Part print with two shaded views. Sizes in mm from the minimum x, y, z corner. Give positions to 0.01 mm unless a question says otherwise; leave off trailing zeros. Write each loop counter-clockwise with the first axis right and the second up, starting at its lowest first coordinate (ties: lowest second). Pieces come first, ordered by that corner, then holes. Notation, with made-up numbers: (-8.5, 74) -> (48.5, 74) arc R27 cw to (48.5, 105) -> close; hole circle Ø3 at (56.5, 49.25). An arc over 180 degrees is marked (long way). Answer as a JSON object with one key per item and string values.
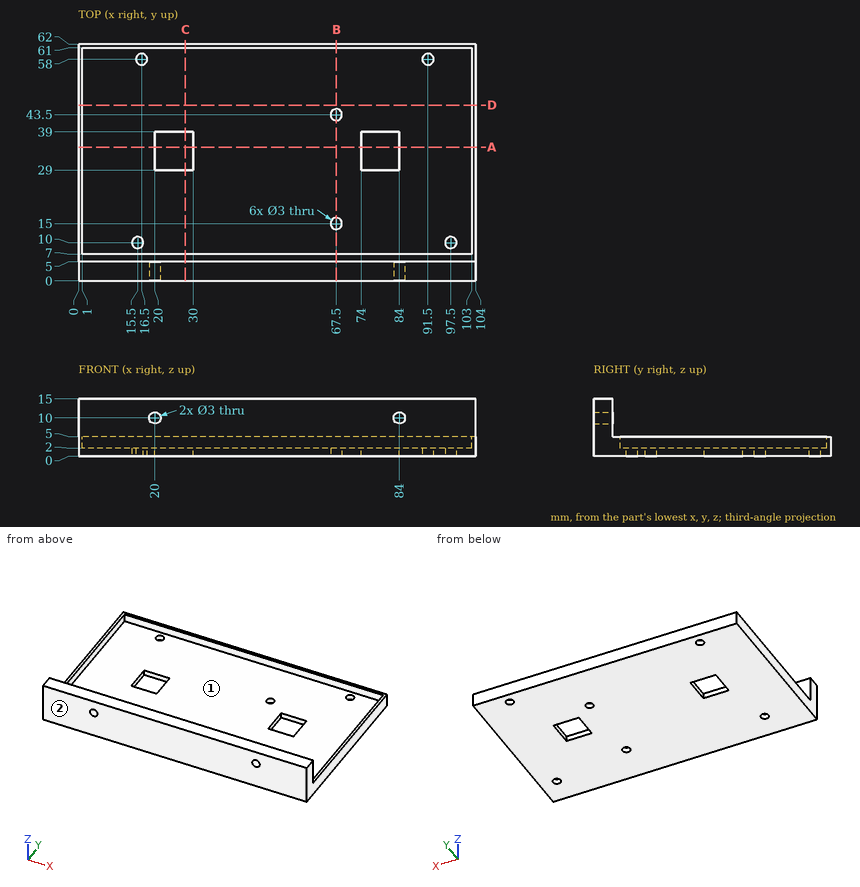
1) Slice it at C-C (x = 28). List the corners of the cut face in (y, z).
Model answer:
{"outline": "(0, 0) -> (29, 0) -> (29, 2) -> (7, 2) -> (7, 5) -> (5, 5) -> (5, 15) -> (0, 15) -> close; (39, 0) -> (62, 0) -> (62, 5) -> (61, 5) -> (61, 2) -> (39, 2) -> close"}
2) Wall check: probe 1 along Y at (x, z) = (67.5, 0.95); probe 2 along Z at (x, y) = (20, 1); probe 3 along X at (y, z) = (43.5, 0.9). Give the ranges that are in metal, low to high.
Model answer:
{"probe 1": "y = 0 to 13.5, 16.5 to 42, 45 to 62", "probe 2": "z = 0 to 8.5, 11.5 to 15", "probe 3": "x = 0 to 66, 69 to 104"}
3) Slice it at A-A (y = 35). List the corners of the cut face in (x, z), then the cut area to 3 significant figures.
Model answer:
{"outline": "(0, 0) -> (20, 0) -> (20, 2) -> (1, 2) -> (1, 5) -> (0, 5) -> close; (30, 0) -> (74, 0) -> (74, 2) -> (30, 2) -> close; (84, 0) -> (104, 0) -> (104, 5) -> (103, 5) -> (103, 2) -> (84, 2) -> close", "area": "174 mm2"}
4) Pin check, flat tips, straight feed: pin 1 (5 mm diameter, centred on x = 25, y = 8, fed in from +Z); pin 2 (3 mm diameter, centred on x = 39, z = 7, fed in from +Y); pin 3 (5 mm diameter, centred on x = 45.5, y = 26, fed in from +Z). Stop position of each tip, or through.
Model answer:
{"pin 1": "stops at z = 5", "pin 2": "stops at y = 5", "pin 3": "stops at z = 2"}
5) Slice it at B-B (x = 67.5). List the corners of the cut face in (y, z).
Model answer:
{"outline": "(0, 0) -> (13.5, 0) -> (13.5, 2) -> (7, 2) -> (7, 5) -> (5, 5) -> (5, 15) -> (0, 15) -> close; (16.5, 0) -> (42, 0) -> (42, 2) -> (16.5, 2) -> close; (45, 0) -> (62, 0) -> (62, 5) -> (61, 5) -> (61, 2) -> (45, 2) -> close"}
6) Mould opens along X. For the marked faces 1 and 2 say: released by +X, released by -X, zero draft, split by the parting line, or undercut.
Model answer:
{"face 1": "undercut", "face 2": "zero draft"}
7) Slice it at D-D (y = 46). List the corners of the cut face in (x, z), then the cut area to 3 significant figures.
Model answer:
{"outline": "(0, 0) -> (104, 0) -> (104, 5) -> (103, 5) -> (103, 2) -> (1, 2) -> (1, 5) -> (0, 5) -> close", "area": "214 mm2"}
